Can you work these out from the drawing? Everything is in mm from the part's minimum corner. Coordinates: 2 decimals unless noted, no trailing zeros. Write each loop counter-clockwise with the first axis right and the second up, starting at its lowest first coordinate (ties: lowest second). Pieces come first, ordered by that corner, then holes. Notation, with made-up numbers: M 44.5,13.5 L 101.5,13.5 A31 ccw 101.5,40.5 Z; hole C -5.75,-31 d8. An arc over 180 degrees is marked long. Answer as a JSON object with one key per item and string values. Group by question number.
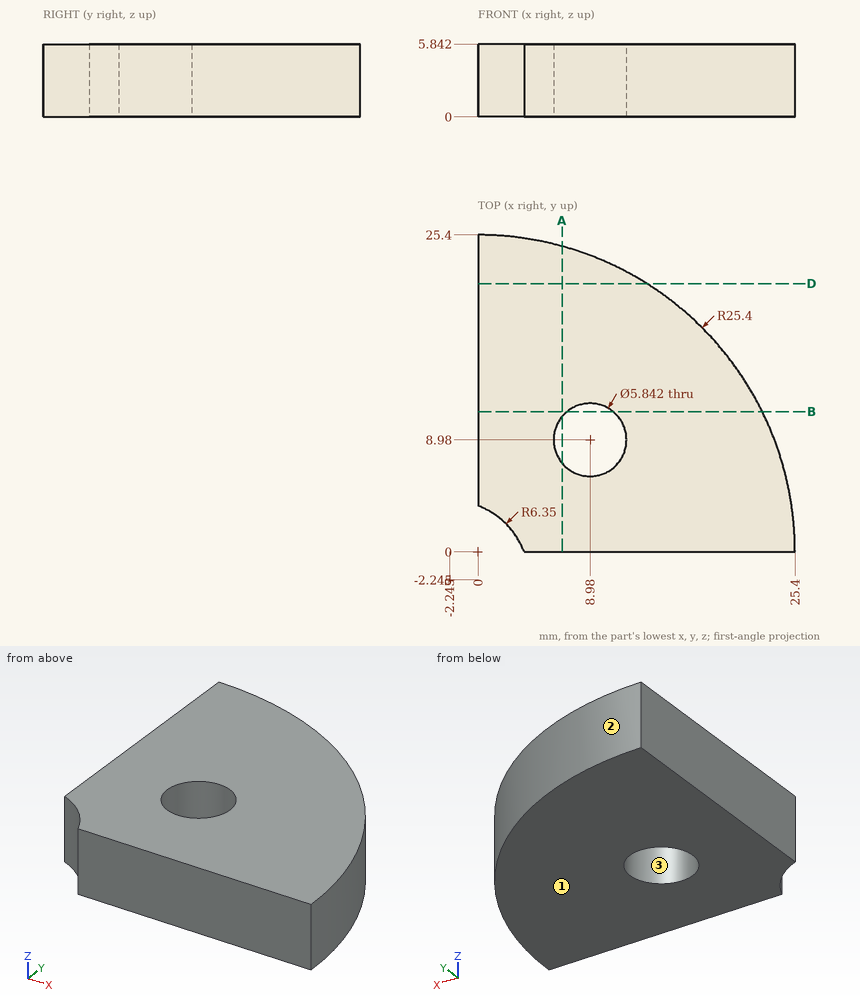
Q1. Please list where these lines run through material, in increasing order: L1, parallel to X at y = 7.5, z = 0.8; L2, parallel to Y at x = 9, z = 2.3; L3, parallel to Y at x = 9.5, z = 2.95 (1 decimal).
Q2. If we section it at D-D on y = 21.5: List the corners of the cut face in (x, z) for me, and give its area (3 significant figures).
Q3. If we section it at B-B on y = 11.25: List the corners of the cut face in (x, z) for me.
Q4. If we section it at A-A on x = 6.75: List the corners of the cut face in (y, z) for me.
Q5. We'd pull the mould along X, two halves only. Please class the marked faces 1, 2 and 3: pulls with the +X half, pulls with the -X half, needs draft (parallel to the pull), parting line crosses it, or undercut.
Q6. Will this pin go through, and if not, where does the flat tip stop? pin 1 (1 mm diameter, centred on y = 2.5, z = 3, fed in from +X).
Reply:
{
 "1": {"L1": "0 to 6.46, 11.5 to 24.27", "L2": "0 to 6.06, 11.9 to 23.75", "L3": "0 to 6.1, 11.9 to 23.6"},
 "2": {"outline": "M 0,0 L 13.52,0 L 13.52,5.84 L 0,5.84 Z", "area": "79.0 mm^2"},
 "3": {"outline": "M 0,0 L 7.14,0 L 7.14,5.84 L 0,5.84 Z; M 10.82,0 L 22.77,0 L 22.77,5.84 L 10.82,5.84 Z"},
 "4": {"outline": "M 0,0 L 7.09,0 L 7.09,5.84 L 0,5.84 Z; M 10.87,0 L 24.49,0 L 24.49,5.84 L 10.87,5.84 Z"},
 "5": {"face 1": "needs draft", "face 2": "pulls with the +X half", "face 3": "undercut"},
 "6": {"pin 1": "x = 25.32"}
}
